Verification items for the finished model (mm, model axes). Coordinates: 2 decimals unless noted, no trailing zeros. Loops run counter-clockwise (first coordinate to the right, second up) from the corner with the lowest first, then second, coordinate; pieces in that order, holes last.
Q1. Mould release check, pull along Y, two halves, no side actions. Record for faces 1 (the face through (-9.859, 1.203, 1.521)), 2 (the face through (9.797, 148.859, 1.521)), 3 (the face through (5.5, 4.07, 1.48)): +Y half, -Y half, draft (parallel to the pull), parting line (faces both ways), or undercut.
Q2. Sectioned sample at A-A (y = 18). Enter the section's corners in (x, z).
Q3. Material ranges on probe 1 along Y at (x, z) = (-7, 2.4); probe 2 along Y at (x, z) = (6.5, 1); probe 3 along X at (y, z) = (17, 0.9), recorded low to high.
```python
from build123d import *

# Parameters (mm, degrees)
ESQUISSE1_W        = 22
ESQUISSE1_H        = 150
ESQUISSE1_R        = 1.5
BOSS_EXTRU_1_DEPTH = 3
CONG_1_R           = 4


with BuildPart() as part:
    # Esquisse1 → Boss.-Extru.1 (new body)
    with BuildSketch(Plane.XY):
        with Locations((0, 75)):
            Rectangle(ESQUISSE1_W, ESQUISSE1_H)
        with Locations((7, 4)):
            Circle(ESQUISSE1_R, mode=Mode.SUBTRACT)
        with Locations(Location((-7, 4, 0), (0, 0, 180))):
            Circle(ESQUISSE1_R, mode=Mode.SUBTRACT)
        with Locations(Location((7, 18, 0), (0, 0, 180))):
            Circle(ESQUISSE1_R, mode=Mode.SUBTRACT)
        with Locations((-7, 18)):
            Circle(ESQUISSE1_R, mode=Mode.SUBTRACT)
    extrude(amount=BOSS_EXTRU_1_DEPTH)

    # Congé1
    cong_1_edges = [part.edges().sort_by_distance(p)[0] for p in [
        (-11, 150, 1.5),
        (11, 150, 1.5),
        (11, 0, 1.5),
        (-11, 0, 1.5),
    ]]
    fillet(cong_1_edges, radius=CONG_1_R)


solid = part.part
```
Geometry check:
1. face 1: -Y half
1. face 2: +Y half
1. face 3: undercut
2. outline: (-11, 0) - (-8.5, 0) - (-8.5, 3) - (-11, 3) - close; (-5.5, 0) - (5.5, 0) - (5.5, 3) - (-5.5, 3) - close; (8.5, 0) - (11, 0) - (11, 3) - (8.5, 3) - close
3. probe 1: y = 0 to 2.5, 5.5 to 16.5, 19.5 to 150
3. probe 2: y = 0 to 2.59, 5.41 to 16.59, 19.41 to 150
3. probe 3: x = -11 to -8.12, -5.88 to 5.88, 8.12 to 11
